Input: part model. Units: mm. Frame: model coordinates. A direction names the side the tool comes from. Coordinates: 2 decimals unless noted, no trailing zeros. Write each loop counter-clockwise with the first axis right and the second up, starting at its lowest first coordinate (ties: lowest second). Pieces come first, ordered by that corner, then holes. Notation, with made-up numbers: (64, 78) - (103, 78) arc R27 ccw to (103, 109) - close; hole circle Ø2 at (-22, 61). An arc over 180 degrees is marked (long way). Use a Markdown table: item, result. Add a question column.
Q1. Pin query (flat end, axial travel): P1, Ø0.5, axis at y = 1, z = 175.5, coming from the +X side; P2, Ø0.5, axis at x = 148.5, y = 1, coming from the -Z side; P3, Ø0.5, axis at y = 0.5, z = 172.5, coming from the -X side. Return the tip coordinate at first contact, or that it passes through.
Q2. Material intervals for probe 1 along Z at (x, y) = (-73.5, 0.95); probe 2 along Z at (x, y) = (-95.5, 1.1); probe 3 along X at (y, z) = (0.55, 140.5), sorted ascending. Write a range as from..to.
Q3. Section query B-B (z = 31.5). Return the cut outline in (x, y), then the cut area to 3 significant figures.
Q4. Section query A-A (x = 59.5). Return the cut outline in (y, z).
Q5. Mould query, pull axis X, two halves, no side actions, for faces 1 (the face through (119.74, 0.8, -36.19)), 2 (the face through (-267.28, 0.8, -36.47)), 3 (the face through (-194.132, 0.805, -162.056)), 4 (the face through (100.184, 0.783, 93.599)). Classes: released by +X, released by -X, zero draft, split by the parting line, or undercut.
Q6. Set-up query: faces 5 (the face through (47.561, 0.805, -162.336)), 6 (the face through (54.78, 0.78, -189.27)). Return all of +Z, -Z, +X, -X, +Y, -Y with unobstructed straight access to the full face (end or side cutting, diameter ignored); none if empty.
Q7. Section query C-C (x = -138.5). Return the cut outline in (y, z), then the cut area to 3 significant figures.
from build123d import *

# Parameters (mm, degrees)
BOSS_EXTRUDE1_DEPTH = 1.5875
SKETCH2_W           = 145.335303163
SKETCH2_H           = 40
CUT_EXTRUDE1_DEPTH  = 1.5875


with BuildPart() as part:
    # Sketch1 → Boss-Extrude1 (new body)
    with BuildSketch(Plane(origin=(0, 0, 0), x_dir=(1, 0, 0), z_dir=(0, 1, 0))):
        Polygon((-186.195305431, -192.980619007), (39.139997732, -192.980619007), (31.222715493, -179.267483912), (36.721976807, -176.092483912), (44.63925905, -189.805619015), (157.306910641, 5.34047791), (141.472346164, 5.34047791), (141.47234615, 11.690477885), (157.306910636, 11.690477885), (44.639259046, 206.83657481), (36.721976807, 193.123439715), (31.222715493, 196.298439715), (39.139997732, 210.01157481), (-186.195305431, 210.01157481), (-178.278023193, 196.298439715), (-183.777284507, 193.123439715), (-191.694566745, 206.83657481), (-304.362218326, 11.690477902), (-288.52765385, 11.690477902), (-288.52765385, 5.340477902), (-304.362218326, 5.340477902), (-191.694566745, -189.805619007), (-183.777284507, -176.092483912), (-178.278023193, -179.267483912), align=None)
        Polygon((-86.22765385, 15.84782632), (-86.22765385, 1.183129483), (-73.52765385, -6.149218936), (-60.82765385, 1.183129483), (-60.82765385, 15.84782632), (-73.52765385, 23.180174739), align=None, mode=Mode.SUBTRACT)
    extrude(amount=BOSS_EXTRUDE1_DEPTH)

    # Sketch2 → Cut-Extrude1 (cut)
    with BuildSketch(Plane(origin=(0, 1.5875, 0), x_dir=(1, 0, 0), z_dir=(0, 1, 0))):
        with Locations((-73.527653849, -172.980619007)):
            Rectangle(SKETCH2_W, SKETCH2_H)
        Polygon((137.306910632, 46.331494061), (64.63925905, 172.195558667), (29.998242899, 152.195558667), (102.66589448, 26.331494061), align=None)
        Polygon((-211.694566745, 172.195558659), (-284.362218326, 46.331494053), (-249.721202175, 26.331494053), (-177.053550594, 152.195558659), align=None)
    extrude(amount=-CUT_EXTRUDE1_DEPTH, mode=Mode.SUBTRACT)


solid = part.part
Values follow:
| question | item | result |
|---|---|---|
| 1 | P1 | x = 53.04 |
| 1 | P2 | z = -27.38 |
| 1 | P3 | x = -201.83 |
| 2 | probe 1 | -210.01..-23.16, 6.13..152.98 |
| 2 | probe 2 | -210.01..152.98 |
| 2 | probe 3 | -220.16..73.11 |
| 3 | outline | (-283.09, 0) - (136.04, 0) - (136.04, 1.59) - (-283.09, 1.59) - close |
| 3 | area | 665 mm2 |
| 4 | outline | (0, -181.1) - (1.59, -181.1) - (1.59, -169.23) - (0, -169.23) - close; (0, -101.1) - (1.59, -101.1) - (1.59, 164.07) - (0, 164.07) - close |
| 5 | face 1 | undercut |
| 5 | face 2 | undercut |
| 5 | face 3 | released by -X |
| 5 | face 4 | released by +X |
| 6 | face 5 | +X, +Y, -Y |
| 6 | face 6 | -Z, +X, +Y, -Y |
| 7 | outline | (0, -210.01) - (1.59, -210.01) - (1.59, 152.98) - (0, 152.98) - close |
| 7 | area | 576 mm2 |
